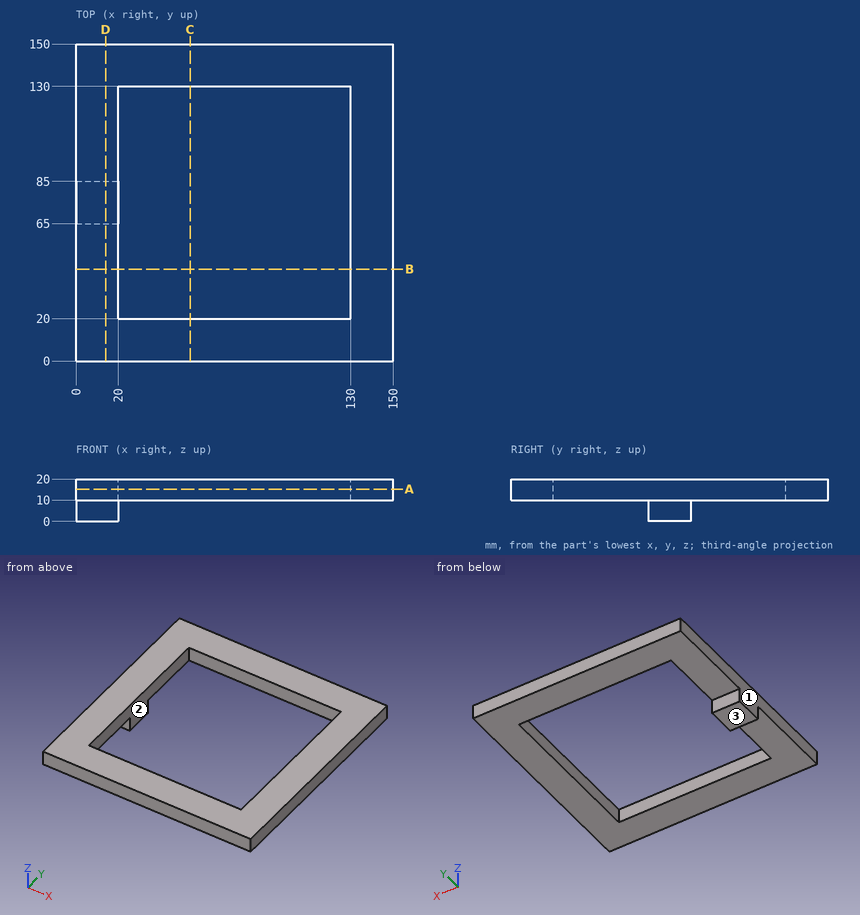
Geometry: see drawing. Coordinates: mm, zero at the bounding-box minimum. Give positions to 0.01 mm unless a question says otherwise; leave off trailing zeros. Write each loop counter-clockwise with the first axis right and the second up, starting at its lowest first coordinate (ties: lowest second). Pieces come first, ordered by that corner, then holes. Notation, with made-up numbers: M 89,14 L 109,14 A21 cw 109,42 Z; hole C 83.5,24 d9. An arc over 180 degrees is marked long. Answer as a JSON object with one key per item and string values.
Q1. Cut plane B-B, the plane y = 43.5. Return the cut outline in (x, z), then the cut area to 3 significant figures.
Geometry check:
{"outline": "M 0,10 L 20,10 L 20,20 L 0,20 Z; M 130,10 L 150,10 L 150,20 L 130,20 Z", "area": "400 mm^2"}
Q2. Mould query, pull axis X, two halves, no side actions, for the marked faces 1, 2 and 3. Classes: +X half, -X half, draft (parallel to the pull), parting line (faces both ways), or undercut.
Geometry check:
{"face 1": "-X half", "face 2": "undercut", "face 3": "draft"}
Q3. Contact query for flat-ended pins moving along their axis: P1, Ø8, axis at x = 10, z = 5, coming from the +Y side; P2, Ø5, axis at x = 15, z = 4, coming from the -Y side. Output: stop coordinate, or through.
Geometry check:
{"P1": "stops at y = 85", "P2": "stops at y = 65"}
Q4. Ray query, line 1 along Y through (x, z) = (46.5, 18.75); line 2 along Z through (x, y) = (73.5, 19). Return the intervals inside material, ascending.
Geometry check:
{"line 1": "y = 0 to 20, 130 to 150", "line 2": "z = 10 to 20"}
Q5. Cut plane A-A, the plane z = 15.25. Return the cut outline in (x, y), then the cut area to 3 significant figures.
Geometry check:
{"outline": "M 0,0 L 150,0 L 150,150 L 0,150 Z; hole M 20,20 L 130,20 L 130,130 L 20,130 Z", "area": "10,400 mm^2"}
Q6. Cut plane D-D, the plane x = 14. Return the cut outline in (y, z), then the cut area to 3 significant figures.
Geometry check:
{"outline": "M 0,10 L 65,10 L 65,0 L 85,0 L 85,10 L 150,10 L 150,20 L 0,20 Z", "area": "1,700 mm^2"}
